Check sheet for the modelled part. Datum: model origin and axes. Units: mm. A direction names the side the tool comes from. Coordinates: 2 decimals unless noted, no trailing zeros. Order: outer loops, then holes, each group sorted by start corner. A loop starts at its lowest first (then second) coordinate and runs counter-clockwise, first axis right, second up.
Autodesk Inventor part; units mm, degrees
ref_plane "YZ Plane" through (0, 0, 0) normal (1, 0, 0) x (0, 1, 0)
ref_plane "XZ Plane" through (0, 0, 0) normal (0, 1, 0) x (-1, 0, 0)
ref_plane "XY Plane" through (0, 0, 0) normal (0, 0, 1) x (1, 0, 0)
sketch "Boceto1" plane through (0, 0, 0) normal (0, 1, 0) x (-1, 0, 0)
  line L0 (0, 10) -> (110, 10)
  line L1 (110, 10) -> (110, -10)
  line L2 (110, -10) -> (0, -10)
  line L3 (0, -10) -> (0, 10)
  line L4 (0, 0) -> (110, 0) construction
  line L5 (68.8, -5) -> (75, -5)
  line L6 (75, -5) -> (75, 5)
  line L7 (75, 5) -> (68.8, 5)
  line L8 (68.8, 5) -> (68.8, -5)
  line L9 (71.9, -5) -> (71.9, -10) construction
  line L10 (71.9, 5) -> (71.9, 10) construction
  line L11 (55, -10) -> (55, 10) construction
  line L12 (41.2, -5) -> (35, -5)
  line L13 (35, -5) -> (35, 5)
  line L14 (35, 5) -> (41.2, 5)
  line L15 (41.2, 5) -> (41.2, -5)
  line L16 (58.6062, -3.6062) -> (51.3938, -3.6062) construction
  line L17 (51.3938, -3.6062) -> (51.3938, 3.6062) construction
  line L18 (51.3938, 3.6062) -> (58.6062, 3.6062) construction
  line L19 (58.6062, 3.6062) -> (58.6062, -3.6062) construction
  circle A0 centre (55, 0) radius 4 construction
  circle A1 centre (55, 0) radius 3.05
  circle A2 centre (55, 0) radius 5.1 construction
  dimension "d28" = 10.2
  dimension "d6" = 110
  dimension "d10" = 10
  dimension "d12" = 5
  dimension "d13" = 20
  dimension "d16" = 6.2
  dimension "d18" = 8
  dimension "d19" = 35
  dimension "d27" = 6.1
extrude "Extrusión1" add sketch "Boceto1" along normal blind 20
sketch "Boceto3" plane through (-110, 0, -10) normal (-1, 0, 0) x (0, 0, 1)
  circle A0 centre (10, 10) radius 3.15
  line L0 (20, 20) -> (0, 20) construction
  line L1 (0, 20) -> (20, 0) construction
  line L2 (0, 0) -> (20, 0) construction
  line L3 (20, 20) -> (0, 0) construction
  point P0 (10, 0)
  dimension "d4" = 6.3
extrude "Extrusión2" cut sketch "Boceto3" against normal up to next
sketch "Boceto5" plane through (-110, 0, -10) normal (-1, 0, 0) x (0, 0, 1)
  circle A0 centre (10, 10) radius 3.15
  circle A1 centre (10, 10) radius 9.1
  point P0 (10, 0)
  dimension "d8" = 18.2
extrude "Extrusión3" cut sketch "Boceto5" against normal blind 2
sketch "Boceto6" plane through (0, 0, 10) normal (1, 0, 0) x (0, 0, -1)
  circle A0 centre (10, 10) radius 3.15
  circle A1 centre (10, 10) radius 9.1
  point P0 (10, 0)
extrude "Extrusión4" cut sketch "Boceto6" against normal up to next contours A0
sketch "Boceto7" plane through (0, 0, 10) normal (1, 0, 0) x (0, 0, -1)
  circle A0 centre (10, 10) radius 9.1
  point P0 (10, 0)
extrude "Extrusión5" cut sketch "Boceto7" against normal blind 2
fillet "Empalme1" radius 7 4 edges at (-55, 0, 10) (-55, 0, -10) (-55, 20, -10) (-55, 20, 10)
(1) Thickness scan on probe 1 along X at (y, z) = (16.75, -4.25); probe 2 along X at (y, z) = (18, -4.75); probe 3 along X at (y, z) = (15.25, 0). Record the ranges inside material, lowest first.
Filled in:
probe 1: x = -108 to -75, -68.8 to -41.2, -35 to -2
probe 2: x = -110 to -75, -68.8 to -41.2, -35 to 0
probe 3: x = -108 to -75, -68.8 to -58.05, -51.95 to -41.2, -35 to -2
(2) Cross-section at D-D (y = 2.5). Enter the section's corners in (x, z), and give its area (3 significant figures).
Filled in:
outline: (-110, -8.36) - (0, -8.36) - (0, -5.15) - (-2, -5.15) - (-2, 5.15) - (0, 5.15) - (0, 8.36) - (-110, 8.36) - (-110, 5.15) - (-108, 5.15) - (-108, -5.15) - (-110, -5.15) - close; hole (-75, -5) - (-68.8, -5) - (-68.8, 5) - (-75, 5) - close; hole circle Ø6.1 at (-55, 0); hole (-41.2, -5) - (-35, -5) - (-35, 5) - (-41.2, 5) - close
area: 1,650 mm2
(3) Tool access check on faces 1 (the flat face through (-108, 10, 4)), 2 (the flat face through (-17, 0, 0)), 3 (the flat face through (-68.8, 10, 0)), 4 (the cylindrical face through (-18.269, 13.123, 0.41)). Record the directions out of +Z, -Z, +X, -X, +Y, -Y that give a thin tool (end or side, any length) a straight path to the whole face; none if there is none.
Filled in:
face 1: -X
face 2: +Z, -Z, +X, -X, -Y
face 3: +Y, -Y
face 4: +X
(4) Release check for a two-part mould opening along X. For faces 5 (the flat face through (-75, 7.6, -2.3)), 6 (the cylindrical face through (-55.8, 18, -7.9)), 7 (the flat face through (0, 18.1, -4.5)) record: +X half, -X half, draft (parallel to the pull), parting line (faces both ways), or undercut.
Filled in:
face 5: undercut
face 6: draft
face 7: +X half
(5) Cross-section at A-A (z = 0). Count the separate pieces of the cut face and the enclosed holes in it, and give its area (3 significant figures).
Filled in:
separate pieces: 6
enclosed holes: 0
area: 1,340 mm2
(6) Go/stop test with flat-tipped pins: P1, Ø3, axis at y = 11, z = 0, coming from the +X side; P2, Ø1, axis at x = -36, z = -3, coming from the +Y side; P3, Ø1, axis at y = 11.5, z = 5.5, coming from the +X side; P4, Ø9, axis at y = 12.5, z = -3.5, coming from the -X side. Record where each tip stops, or that it passes through.
Filled in:
P1: stops at x = -41.2
P2: passes through
P3: stops at x = -2
P4: stops at x = -108
(7) Cross-section at C-C (x = -47.5). Enter the section's corners in (y, z), and give its area (3 significant figures).
Filled in:
outline: (0, -3) arc R7 ccw to (7, -10) - (13, -10) arc R7 ccw to (20, -3) - (20, 3) arc R7 ccw to (13, 10) - (7, 10) arc R7 ccw to (0, 3) - close
area: 358 mm2
